For this review, take the finished solid that the model builds, in its own axes (mm). Give positions to 0.01 mm unless a question says otherwise; leave off trailing zeros. Order: outer loops, then holes, each group sorted by start corner. A loop starts at its lowest first (then second) coordinate and runs counter-clockwise, first axis right, second up.
from build123d import *

# Parameters (mm, degrees)
SKETCH_1_R          = 15
EXTRUDE_5_DEPTH     = 3
SKETCH_8_R          = 16
EXTRUDE_7_DEPTH     = 1
SKETCH_9_R          = 7.5
CUT_EXTRUDE_3_DEPTH = 9
HOLE_WIZARD_M3_1_D  = 2.5
CHAMFER_1_SIZE      = 0.3
CHAMFER_2_SIZE      = 0.3


with BuildPart() as part:
    # 草图1 → 凸台-拉伸5 (new body)
    with BuildSketch(Plane.XY):
        Circle(SKETCH_1_R)
    extrude(amount=EXTRUDE_5_DEPTH)

    # 草图8 → 凸台-拉伸7 (add)
    with BuildSketch(Plane(origin=(0, 0, 0), x_dir=(-1, 0, 0), z_dir=(0, 0, -1))):
        Circle(SKETCH_8_R)
    extrude(amount=-EXTRUDE_7_DEPTH)

    # 草图9 → 切除-拉伸3 (cut)
    with BuildSketch(Plane(origin=(0, 0, 0), x_dir=(-1, 0, 0), z_dir=(0, 0, -1))):
        Circle(SKETCH_9_R)
    extrude(amount=-CUT_EXTRUDE_3_DEPTH, mode=Mode.SUBTRACT)

    # M3 螺纹孔1 (through all)
    with Locations(Plane(origin=(0, 0, 0), x_dir=(-1, 0, 0), z_dir=(0, 0, -1))):
        with Locations((0, 0), (0, 12), (10.392304845, 6), (10.392304845, -6), (0, -12), (-10.392304845, -6), (-10.392304845, 6)):
            Hole(HOLE_WIZARD_M3_1_D / 2)

    # 倒角1
    chamfer_1_edges = [part.edges().sort_by_distance(p)[0] for p in [
        (-15, 0, 3),
    ]]
    chamfer(chamfer_1_edges, length=CHAMFER_1_SIZE)

    # 倒角2
    chamfer_2_edges = [part.edges().sort_by_distance(p)[0] for p in [
        (7.5, 0, 3),
    ]]
    chamfer(chamfer_2_edges, length=CHAMFER_2_SIZE)


solid = part.part
1) We need section A-A on x = 0. Give the boundary of the cut face in (y, z), then the cut area to 3 significant figures.
Answer sheet:
outline: (-16, 0) - (-13.25, 0) - (-13.25, 3) - (-14.7, 3) - (-15, 2.7) - (-15, 1) - (-16, 1) - close; (-10.75, 0) - (-7.5, 0) - (-7.5, 2.7) - (-7.8, 3) - (-10.75, 3) - close; (7.5, 0) - (10.75, 0) - (10.75, 3) - (7.8, 3) - (7.5, 2.7) - close; (13.25, 0) - (16, 0) - (16, 1) - (15, 1) - (15, 2.7) - (14.7, 3) - (13.25, 3) - close
area: 31.8 mm2
2) To check wall thickness, follow line 1 (Y direction, x = -9.5, z = 1.6); line 2 (Y direction, x = -2.5, z = 1.45); line 3 (Y direction, x = -1.5, z = 2.6). State the ranges of each line that lie inside material, in increasing order.
Answer sheet:
line 1: y = -11.61 to -6.88, -5.12 to 5.12, 6.88 to 11.61
line 2: y = -14.79 to -7.07, 7.07 to 14.79
line 3: y = -14.92 to -7.35, 7.35 to 14.92
3) We need section C-C on y = 0. Give the boundary of the cut face in (x, z), then the cut area to 3 significant figures.
Answer sheet:
outline: (-16, 0) - (-7.5, 0) - (-7.5, 2.7) - (-7.8, 3) - (-14.7, 3) - (-15, 2.7) - (-15, 1) - (-16, 1) - close; (7.5, 0) - (16, 0) - (16, 1) - (15, 1) - (15, 2.7) - (14.7, 3) - (7.8, 3) - (7.5, 2.7) - close
area: 46.8 mm2
4) Draft analysis for pull direction X (two halves, no side actions). For faces 1 (the face through (-0.16, 13.24, 1.52)), 2 (the face through (-14.985, 0.66, 1.838)), 3 (the face through (6, -6, 3)), state which applies: +X half, -X half, draft (parallel to the pull), parting line (faces both ways), or undercut.
Answer sheet:
face 1: undercut
face 2: parting line
face 3: draft
5) We need section D-D on y = 6. Count the separate pieces of the cut face and the enclosed holes in it, then the cut area to 3 significant figures.
Answer sheet:
separate pieces: 4
enclosed holes: 0
area: 42.4 mm2
6) We need section B-B on z = 1.8. Give the boundary of the cut face in (x, y), then the cut area to 3 significant figures.
Answer sheet:
outline: circle Ø30 at (0, 0); hole circle Ø2.5 at (-10.39, -6); hole circle Ø2.5 at (-10.39, 6); hole circle Ø15 at (0, 0); hole circle Ø2.5 at (0, -12); hole circle Ø2.5 at (0, 12); hole circle Ø2.5 at (10.39, -6); hole circle Ø2.5 at (10.39, 6)
area: 501 mm2
